Input: part model. Units: mm. Frame: model coordinates. Round coordinates to 2 decimals unless told otherwise and drop trailing zeros. Loops run counter-clockwise (first coordinate to the right, second up) from the corner with the lowest first, then second, coordinate; pieces in that order, holes last. Notation, with made-up numbers: (-23.75, 32) -> (15.25, 32) arc R19 ccw to (15.25, 47) -> close; hole circle Ø2 at (12, 68.5). An arc over 180 degrees is marked (long way). Answer in a Markdown table with one row per item. Add a question column.
Q1. Section C-C, the plane z = 17. Output: boundary loops of the cut face in (x, y).
Q2. Section B-B, the plane x = 5. Output: boundary loops of the cut face in (y, z), and give its area (3 significant figures).
Q3. Pin query (flat end, axial travel): pin 1 (1.3 mm diameter, centred on y = 1, z = -40, fed in from -X); pin 2 (1 mm diameter, centred on x = -9, y = 1, fed in from -Z); pin 3 (0.8 mm diameter, centred on y = 1.5, z = -16, fed in from +X). Return the tip coordinate at first contact, or that it passes through.
Q4. Section A-A, the plane y = 1.15. Output: boundary loops of the cut face in (x, z).
Q5. Ray query, L1, parallel to Z at x = -11, y = 2.3; L2, parallel to X at y = 0.95, z = 13; L3, parallel to Z at x = 7.5, y = 1.45. Return the intervals inside material, ascending. Write a range as from..to.
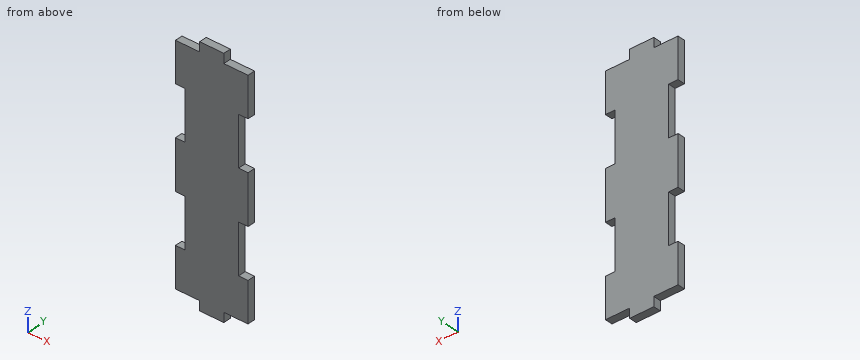
```python
from build123d import *

# Parameters (mm, degrees)
SKETCH1_W           = 24.384
SKETCH1_H           = 83.185
BOSS_EXTRUDE1_DEPTH = 2.54
SKETCH2_W           = 3.175
SKETCH2_H           = 16.637
CUT_EXTRUDE1_DEPTH  = 2.54
LPATTERN1_COUNT     = 2
LPATTERN1_PITCH     = 33.274
SKETCH3_W           = 8.128
SKETCH3_H           = 3.175
CUT_EXTRUDE5_DEPTH  = 3.175
LPATTERN3_COUNT     = 2
LPATTERN3_PITCH     = 16.256


with BuildPart() as part:
    # Sketch1 → Boss-Extrude1 (new body)
    with BuildSketch(Plane(origin=(0, 0, 0), x_dir=(1, 0, 0), z_dir=(0, 1, 0))):
        Rectangle(SKETCH1_W, SKETCH1_H)
    extrude(amount=BOSS_EXTRUDE1_DEPTH)

    # Sketch2 → Cut-Extrude1 (cut)
    with BuildSketch(Plane(origin=(0, 2.54, 0), x_dir=(1, 0, 0), z_dir=(0, 1, 0))):
        with Locations((-10.6045, 16.637)):
            Rectangle(SKETCH2_W, SKETCH2_H)
        with Locations((10.6045, 16.637)):
            Rectangle(SKETCH2_W, SKETCH2_H)
    cut_extrude1 = extrude(amount=-CUT_EXTRUDE1_DEPTH, mode=Mode.SUBTRACT)

    # LPattern1: Cut-Extrude1 ×2
    with Locations(*[(0, 0, i * LPATTERN1_PITCH) for i in range(1, LPATTERN1_COUNT)]):
        add(cut_extrude1, mode=Mode.SUBTRACT)

    # Sketch3 → Cut-Extrude5 (cut)
    with BuildSketch(Plane(origin=(0, 2.54, 0), x_dir=(1, 0, 0), z_dir=(0, 1, 0))):
        with Locations((8.128, 40.005)):
            Rectangle(SKETCH3_W, SKETCH3_H)
        with Locations((8.128, -40.005)):
            Rectangle(SKETCH3_W, SKETCH3_H)
    cut_extrude5 = extrude(amount=-CUT_EXTRUDE5_DEPTH, mode=Mode.SUBTRACT)

    # LPattern3: Cut-Extrude5 ×2
    with Locations(*[(-i * LPATTERN3_PITCH, 0, 0) for i in range(1, LPATTERN3_COUNT)]):
        add(cut_extrude5, mode=Mode.SUBTRACT)


solid = part.part
```
Answer block:
| question | item | result |
|---|---|---|
| 1 | outline | (-9.02, 0) -> (9.02, 0) -> (9.02, 2.54) -> (-9.02, 2.54) -> close |
| 2 | outline | (0, -38.42) -> (2.54, -38.42) -> (2.54, 38.42) -> (0, 38.42) -> close |
| 2 | area | 195 mm^2 |
| 3 | pin 1 | x = -4.06 |
| 3 | pin 2 | z = -38.42 |
| 3 | pin 3 | x = 9.02 |
| 4 | outline | (-12.19, -38.42) -> (-4.06, -38.42) -> (-4.06, -41.59) -> (4.06, -41.59) -> (4.06, -38.42) -> (12.19, -38.42) -> (12.19, -24.96) -> (9.02, -24.96) -> (9.02, -8.32) -> (12.19, -8.32) -> (12.19, 8.32) -> (9.02, 8.32) -> (9.02, 24.96) -> (12.19, 24.96) -> (12.19, 38.42) -> (4.06, 38.42) -> (4.06, 41.59) -> (-4.06, 41.59) -> (-4.06, 38.42) -> (-12.19, 38.42) -> (-12.19, 24.96) -> (-9.02, 24.96) -> (-9.02, 8.32) -> (-12.19, 8.32) -> (-12.19, -8.32) -> (-9.02, -8.32) -> (-9.02, -24.96) -> (-12.19, -24.96) -> close |
| 5 | L1 | -38.42..-24.96, -8.32..8.32, 24.96..38.42 |
| 5 | L2 | -9.02..9.02 |
| 5 | L3 | -38.42..38.42 |
